Read the model definition and answer for the solid it produces. Units are mm, in the model's axes. Face numbers are marked on the shaded views. A direction names the side the tool comes from. Give positions to 0.01 mm unless a question says otherwise; leave off trailing zeros. Order: outer loops, then holes, each group sorted by start corner. A loop starts at its lowest first (then second) coordinate and runs counter-clockwise, first axis right, second up. Notation, with made-up numbers: (51, 28.5) - (73, 28.5) arc R16 ccw to (73, 55.5) - close; hole circle Ø1 at (-28.75, 66.25). An arc over 180 degrees is marked (long way). Write each question's results on one line, items separated by ' | '. Start each with the question number.
Q1. A tool of negligible diameter and unlimited length cuts with its end or side. For the marked faces 1, 2 and 3, from which of +Z, -Z, +X, -X, +Y, -Y can it reach the whole face along a straight path? Write none if from no direction.
Q2. Find section A-A on z = 0. Count the separate pieces of the cut face and the enclosed holes in it, and give its area (3 significant figures).
Q3. Flat-ended cylindrical pins translate along their axes: P1, Ø1.6, axis at x = -1.5, z = -1, coming from the -Y side; P2, Ø2.5, axis at x = -7, z = -1, coming from the -Y side; P3, Ø1.4, axis at x = -3.5, y = -6, coming from the +Z side. Find the tip coordinate at first contact, or state that the pin passes through.
Q4. Find the intervals of material crossed by line 1 along X through (y, z) = (0.45, 0); line 2 along Z through (x, y) = (-7.5, 0.3); line 3 along Y through (x, z) = (-3.75, -0.65), in increasing order. Write a range as from..to.
Q5. Find section C-C on x = -1.25. Give the vertices of the cut face in (y, z).
Q6. Find section D-D on y = 2.75. Give the vertices of the cut face in (x, z).
Q7. Find section B-B on x = 7.5. Give the vertices of the cut face in (y, z).
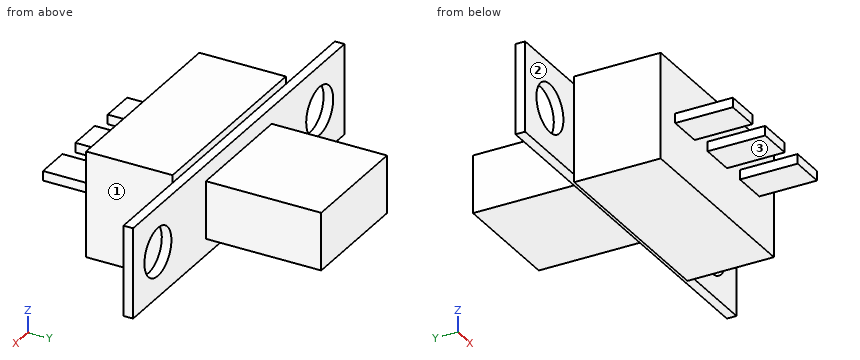
from build123d import *

# Parameters (mm, degrees)
SKETCH_1_W           = 9.8
SKETCH_1_H           = 4.7
SKETCH_1_R           = 1.25
EXTRUDE_1_DEPTH      = 0.5
SKETCH_2_W           = 5.25
SKETCH_2_H           = 5.5
EXTRUDE_2_DEPTH      = 4.5
EXTRUDE_3_DEPTH      = 0.25
EXTRUDE_3_DEPTH_BACK = 0.25
SKETCH_3_W           = 1.8
SKETCH_3_H           = 3
SKETCH_3_W_2         = 0.9
SKETCH_4_W           = 6.1
SKETCH_4_H           = 3
EXTRUDE_4_DEPTH      = 6


with BuildPart() as part:
    # 草图1 → 凸台-拉伸1 (new body)
    with BuildSketch(Plane(origin=(0, 0, 0), x_dir=(1, 0, 0), z_dir=(0, 1, 0))):
        with Locations((4.9, 0)):
            Rectangle(SKETCH_1_W, SKETCH_1_H)
        with Locations(Location((7.5, 0, 0), (0, 0, 270))):
            Circle(SKETCH_1_R, mode=Mode.SUBTRACT)
    extrude(amount=EXTRUDE_1_DEPTH)

    # 草图2 → 凸台-拉伸2 (add)
    with BuildSketch(Plane.XZ):
        with Locations((2.625, 0)):
            Rectangle(SKETCH_2_W, SKETCH_2_H)
    extrude(amount=EXTRUDE_2_DEPTH)

    # 草图3 → 凸台-拉伸3 (add, two sides: drawn at the far end of the back side and taken through both)
    with BuildSketch(Plane.XY.offset(-EXTRUDE_3_DEPTH_BACK)):
        with Locations((3, -6)):
            Rectangle(SKETCH_3_W, SKETCH_3_H)
        with Locations((0.45, -6)):
            Rectangle(SKETCH_3_W_2, SKETCH_3_H)
    extrude(amount=EXTRUDE_3_DEPTH + EXTRUDE_3_DEPTH_BACK)

    # 镜向1: part across plane


with BuildPart() as part_1:
    add(part.part)
    add(part.part.mirror(Plane(origin=(0, 0.5, -2.35), x_dir=(0, 0, 1), z_dir=(1, 0, 0))))

    # 草图4 → 凸台-拉伸4 (add)
    with BuildSketch(Plane(origin=(0, 0.5, 0), x_dir=(1, 0, 0), z_dir=(0, 1, 0))):
        Rectangle(SKETCH_4_W, SKETCH_4_H)
    extrude(amount=EXTRUDE_4_DEPTH)


solid = part_1.part
Working result:
1) face 1: +Z, -Z, +X, -Y | face 2: +Z, -Z, -X, -Y | face 3: -Z, +X, -X, -Y
2) separate pieces: 3 | enclosed holes: 0 | area: 107 mm²
3) P1: y = -4.5 | P2: y = 0 | P3: z = 0.25
4) line 1: -9.8..-8.75, -6.25..6.25, 8.75..9.8 | line 2: -2.35..-1.25, 1.25..2.35 | line 3: -4.5..0.5
5) outline: (-4.5, -2.75) - (0, -2.75) - (0, -2.35) - (0.5, -2.35) - (0.5, -1.5) - (6.5, -1.5) - (6.5, 1.5) - (0.5, 1.5) - (0.5, 2.35) - (0, 2.35) - (0, 2.75) - (-4.5, 2.75) - close
6) outline: (-3.05, -1.5) - (3.05, -1.5) - (3.05, 1.5) - (-3.05, 1.5) - close
7) outline: (0, -2.35) - (0.5, -2.35) - (0.5, -1.25) - (0, -1.25) - close; (0, 1.25) - (0.5, 1.25) - (0.5, 2.35) - (0, 2.35) - close
